The model under review builds one solid part; all positions refer to its coordinate system, in mm. Face numbers are marked on the shaded views. A direction names the side the tool comes from. Round coordinates to 2 decimals unless told otherwise and drop trailing zeros. Answer as a JSON object with one key per item and string values. Group by question number.
1. Clearance check with flat-ended pins moving along their axes: P1, Ø1.3, axis at x = 0, z = 3, coming from the -Y side; P2, Ø1.4, axis at x = -28, z = 2, coming from the +Y side; P3, Ø5, axis at x = 14.5, y = 35, coming from the -Z side; P4, Ø1.4, axis at x = 9, z = 1, coming from the -Y side. State where each tip first meets the part, or that it passes through.
2. Add section A-A on z = 2.25. Give the number of separate pieces and of enclosed holes in the cut face, and give its area (3 significant figures).
3. To check wall thickness, follow probe 1 along Y at (x, z) = (4.5, 1.6); probe 2 along Y at (x, z) = (-30, 3); probe 3 along X at (y, z) = (7, 4.2). State the ranges of each line that lie inside material, in increasing order. Write a range as [from, to].
4. Machinability: for the marked faces 5, 6, 7 and 8, which of the approach directions +Z, -Z, +X, -X, +Y, -Y give a long, thin tool a straight path to every point of the face, cutting with its end or side? Answer none if there is none.
5. Mouldability with a two-part tool opening along Y and no side actions: class the marked faces 1, 2, 3 and 4 as released by +Y, released by -Y, zero draft, split by the parting line, or undercut.
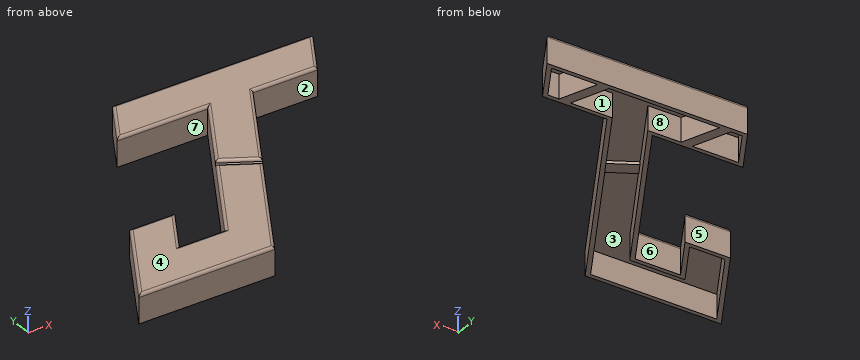
```python
from build123d import *

# Parameters (mm, degrees)
F1_DEPTH = 5
F4_W     = 1
F4_H     = 5.3799478337
F5_DEPTH = 100
F6_T     = -0.75
F7_R     = 0.49999
F9_DEPTH = 4.25


# Not quite as in the source:
# - a fillet or chamfer is up to 0.001 mm smaller than in the source, because OpenCascade refuses the exact size


with BuildPart() as f1:
    # F0 (on Top) → F1 (new body)
    with BuildSketch(Plane.XY):
        Polygon((-15.3811978465, 38), (-20, 30), (-4, 30), (-21.3205080757, 0), (-29.3205080757, 0), (-24.7017059222, 8), (-32.7017059222, 8), (-41.9393102292, -8), (-17.9393102292, -8), (4, 30), (15.3811978465, 30), (20, 38), align=None)
    extrude(amount=F1_DEPTH)

    # F4 (on offset) → F5 (cut)
    with BuildSketch(Plane(origin=(11.6602540378, -6.7320508076, 0), x_dir=(0.5, 0.8660254038, 0), z_dir=(0.8660254038, -0.5, 0))):
        with Locations((8.2942286341, 7.1899739169)):
            Rectangle(F4_W, F4_H)
    extrude(amount=-F5_DEPTH, mode=Mode.SUBTRACT)

    # F6
    f6_openings = [f1.faces().sort_by_distance(p)[0] for p in [
        (2.309401, 37.228477, 0),
    ]]
    offset(amount=F6_T, openings=f6_openings, kind=Kind.INTERSECTION)

    # F7 (radius 0.5 in the source; OpenCascade refuses exactly that, so slightly less here)
    f7_edges = [f1.edges().sort_by_distance(p)[0] for p in [
        (-0.796633, 21.691987, 5),
        (9.690599, 30, 5),
        (17.690599, 34, 5),
        (2.309401, 38, 5),
        (-17.690599, 34, 5),
        (-12, 30, 5),
        (-7.796633, 23.424038, 5),
        (-8.593267, 15.116025, 5),
        (-16.706887, 7.991025, 5),
        (-25.320508, 0, 5),
        (-27.011107, 4, 5),
        (-28.701706, 8, 5),
        (-37.320508, 0, 5),
        (-29.93931, -8, 5),
        (-12.016288, 2.258975, 5),
        (-9.093267, 14.25, 5),
    ]]
    fillet(f7_edges, radius=F7_R)

    # F8 (on face) → F9 (join, through all)
    with BuildSketch(Plane(origin=(0, 0, 4.25), x_dir=(1, 0, 0), z_dir=(0, 0, -1))):
        Polygon((-10.5823786219, -30.75), (-12.9481851446, -37.25), (-10.9481851446, -37.25), (-8.5823786219, -30.75), align=None)
        Polygon((10.9481851446, -30.75), (8.5823786219, -37.25), (10.5823786219, -37.25), (12.9481851446, -30.75), align=None)
    extrude(amount=F9_DEPTH)


solid = f1.part
```
Recorded:
{
 "1": {"P1": "stops at y = 21.95", "P2": "stops at y = 8", "P3": "stops at z = 0", "P4": "stops at y = 30"},
 "2": {"separate pieces": "1", "enclosed holes": "3", "area": "194 mm²"},
 "3": {"probe 1": "y = [30, 30.75], [37.25, 38]", "probe 2": "y = [-8, -7.25], [-0.75, 0.32], [7.25, 8]", "probe 3": "x = [-33.28, -32.41], [-26.15, -25.28], [-17.28, -16.41], [-10.15, -9.28]"},
 "4": {"face 5": "+Z, -Z, -X, +Y", "face 6": "+Z, -Z", "face 7": "+Z, -Z, -X", "face 8": "-Z"},
 "5": {"face 1": "undercut", "face 2": "released by -Y", "face 3": "undercut", "face 4": "zero draft"}
}
